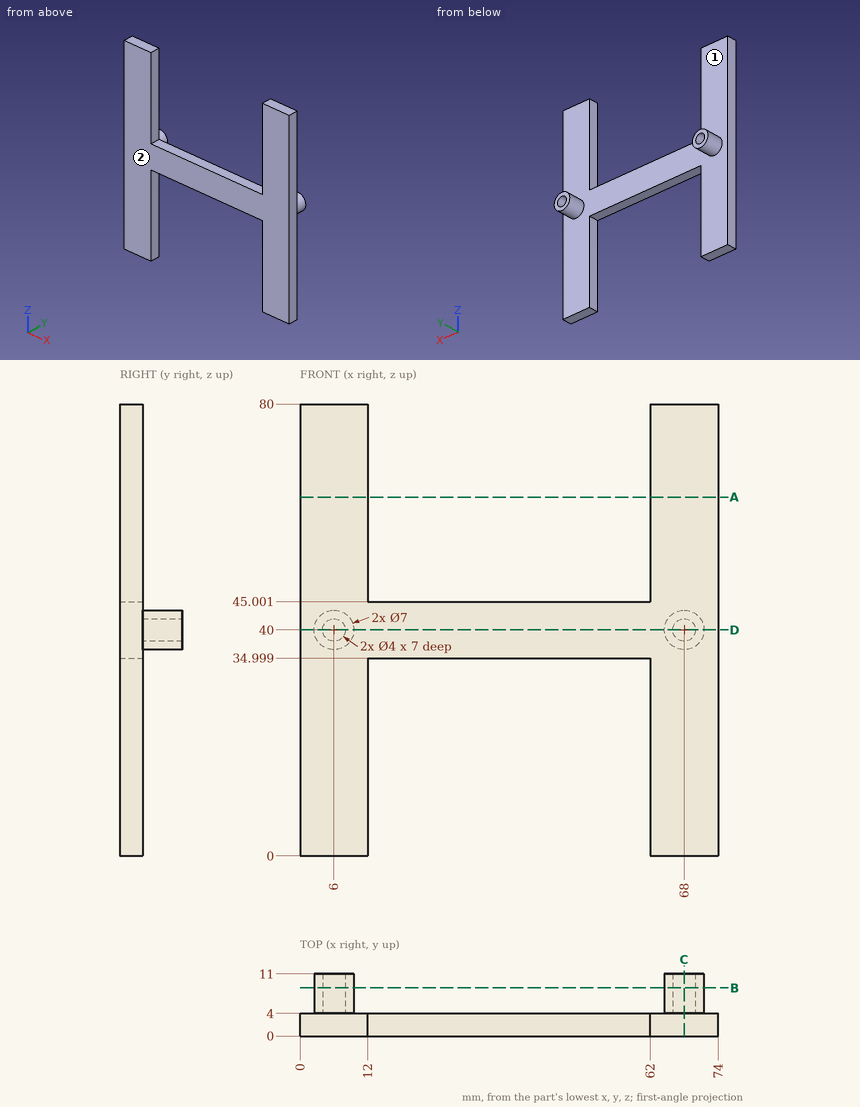
Study the drawing (mm; zero at the part's minimum x, y, z) and answer. Give positions to 0.01 mm unless a question says otherwise; leave off trailing zeros. Write each loop counter-clockwise with the first axis right and the second up, starting at its lowest first coordinate (ties: lowest second). Pieces come first, ordered by that corner, then holes. Notation, with made-up numbers: (-9, -5.75) -> (49, -5.75) arc R12 ccw to (49, 11.25) -> close; hole circle Ø1 at (9.25, 10.5). An arc over 180 degrees is marked (long way). Write item = value, one per line. Start each with the question number.
1) Each of these flat-tipped pins is pushed along its axis until it touches: pin 1 (2 mm diameter, centred on x = 40.5, y = 3, fed in from -Z); pin 2 (1.2 mm diameter, centred on x = 38, y = 2, fed in from +Z); pin 3 (6 mm diameter, centred on x = 58, z = 50, fed in from -Y). Where does it stop, or does it pass through?
2) The part is cut by section B-B, the plane y = 8.5. Determine the outline of the cut face in (x, z).
3) The part is cut by section D-D, the plane z = 40. Determine the outline of the cut face in (x, y), and give its area (3 significant figures).
4) Determine the mould class of the marked faces 1 and 2 for opening direction X: +X half, -X half, draft (parallel to the pull), parting line (faces both ways), or undercut.
5) The part is cut by section A-A, the plane z = 63.5. Determine the outline of the cut face in (x, y).
6) Straight lines are drawn through the part: line 1 along X through (y, z) = (5.5, 40); line 2 along Z through (x, y) = (68, 8.5); line 3 along X through (y, z) = (1.75, 56.5). For each, find the intervals that lie inside material, in ascending order.
7) The part is cut by section C-C, the plane x = 68. Determine the outline of the cut face in (y, z).
Solutions:
q1.pin_1 = 35
q1.pin_2 = 45
q1.pin_3 = through
q2.outline = circle Ø7 at (6, 40); circle Ø7 at (68, 40); hole circle Ø4 at (6, 40); hole circle Ø4 at (68, 40)
q3.outline = (0, 0) -> (74, 0) -> (74, 4) -> (71.5, 4) -> (71.5, 11) -> (70, 11) -> (70, 4) -> (66, 4) -> (66, 11) -> (64.5, 11) -> (64.5, 4) -> (9.5, 4) -> (9.5, 11) -> (8, 11) -> (8, 4) -> (4, 4) -> (4, 11) -> (2.5, 11) -> (2.5, 4) -> (0, 4) -> close
q3.area = 338 mm²
q4.face_1 = undercut
q4.face_2 = draft
q5.outline = (0, 0) -> (12, 0) -> (12, 4) -> (0, 4) -> close; (62, 0) -> (74, 0) -> (74, 4) -> (62, 4) -> close
q6.line_1 = 2.5 to 4, 8 to 9.5, 64.5 to 66, 70 to 71.5
q6.line_2 = 36.5 to 38, 42 to 43.5
q6.line_3 = 0 to 12, 62 to 74
q7.outline = (0, 0) -> (4, 0) -> (4, 36.5) -> (11, 36.5) -> (11, 38) -> (4, 38) -> (4, 42) -> (11, 42) -> (11, 43.5) -> (4, 43.5) -> (4, 80) -> (0, 80) -> close
